Autodesk Inventor part; units mm, degrees
ref_plane "YZ Plane" through (0, 0, 0) normal (1, 0, 0) x (0, 1, 0)
ref_plane "XZ Plane" through (0, 0, 0) normal (0, 1, 0) x (-1, 0, 0)
ref_plane "XY Plane" through (0, 0, 0) normal (0, 0, 1) x (1, 0, 0)
sketch "Sketch1" plane through (0, 0, 0) normal (0, 1, 0) x (-1, 0, 0)
  line L0 (30.48, 38.1) -> (-30.48, 38.1)
  line L1 (-30.48, 38.1) -> (-30.48, -38.1)
  line L2 (-30.48, -38.1) -> (30.48, -38.1)
  line L3 (30.48, -38.1) -> (30.48, 38.1)
  point P0 (0, 0)
  dimension "d0" = 76.2
  dimension "d1" = 60.96
  dimension "d2" = 38.1
  dimension "d3" = 30.48
extrude "Extrusion1" add sketch "Sketch1" along normal blind 25.4
sketch "Sketch2" plane through (0, 25.4, 0) normal (0, 1, 0) x (1, 0, 0)
  line L0 (-28.8925, 36.5125) -> (28.8925, 36.5125)
  line L1 (28.8925, 36.5125) -> (28.8925, -36.5125)
  line L2 (28.8925, -36.5125) -> (-28.8925, -36.5125)
  line L3 (-28.8925, -36.5125) -> (-28.8925, 36.5125)
  point P0 (0, 0)
  dimension "d6" = 73.025
  dimension "d7" = 57.785
  dimension "d8" = 36.5125
  dimension "d9" = 28.8925
extrude "Extrusion2" cut sketch "Sketch2" against normal blind 19.05
chamfer "Chamfer1" distance 0.7937 angle 45 8 edges at (0, 0, 38.1) (30.48, 0, 0) (0, 0, -38.1) (-30.48, 0, 0) (30.48, 12.7, 38.1) (-30.48, 12.7, 38.1) (30.48, 12.7, -38.1) (-30.48, 12.7, -38.1)
sketch "Sketch3" plane through (0, 6.35, 0) normal (0, 1, 0) x (1, 0, 0)
  circle A0 centre (-22.86, 30.48) radius 1.9304
  circle A1 centre (22.86, 30.48) radius 1.9304
  circle A2 centre (-22.86, -30.48) radius 1.9304
  circle A3 centre (22.86, -30.48) radius 1.9304
  line L0 (-28.8925, -36.5125) -> (-28.8925, 36.5125)
  line L1 (-28.8925, 36.5125) -> (28.8925, 36.5125)
  line L2 (0, 0) -> (0, 32.9664)
  line L3 (0, 0) -> (-24.0434, 0)
  line L4 (0, 0) -> (25.6064, 0)
  line L5 (0, 0) -> (0, -31.6413)
  dimension "d15" = 3.8608
  dimension "d16" = 3.8608
  dimension "d17" = 3.8608
  dimension "d18" = 3.8608
  dimension "d21" = 30.48
  dimension "d22" = 22.86
  dimension "d23" = 22.86
  dimension "d24" = 30.48
  dimension "d25" = 22.86
  dimension "d26" = 30.48
  dimension "d27" = 22.86
  dimension "d28" = 30.48
extrude "Extrusion3" cut sketch "Sketch3" against normal blind 6.35
sketch "Sketch4" plane through (0, 0, 0) normal (0, -1, 0) x (1, 0, 0)
  circle A0 centre (-22.86, 30.48) radius 5.08
  line L0 (0, 0) -> (-26.2361, 0)
  line L1 (-26.2361, 0) -> (0, 0)
  line L2 (0, 0) -> (0, 35.0708)
  line L3 (0, 0) -> (27.0223, 0)
  line L4 (0, 0) -> (0, -33.193)
  circle A1 centre (22.86, 30.48) radius 5.08
  circle A2 centre (-22.86, -30.48) radius 5.08
  circle A3 centre (22.86, -30.48) radius 1.9304
  circle A4 centre (22.86, -30.48) radius 5.08
  dimension "d31" = 10.16
  dimension "d32" = 22.86
  dimension "d33" = 30.48
  dimension "d34" = 10.16
  dimension "d35" = 22.86
  dimension "d36" = 30.48
  dimension "d37" = 10.16
  dimension "d38" = 10.16
  dimension "d39" = 30.48
  dimension "d40" = 22.86
extrude "Extrusion4" cut sketch "Sketch4" against normal blind 3.175
properties part number "Enclosure Rev A"
Check sheet for the modelled part. Datum: model origin and axes. Units: mm. A direction names the side the tool comes from. Coordinates: 2 decimals unless noted, no trailing zeros. Loops run counter-clockwise (first coordinate to the right, second up) from the corner with the lowest first, then second, coordinate; pieces in that order, holes last. Notation, with made-up numbers: (33.5, 50.5) -> (70.5, 50.5) arc R20 cw to (70.5, 82.5) -> close; hole circle Ø8 at (-1.5, -7). An arc over 180 degrees is marked (long way). Write item = value, one per line. Start each with the question number.
1. Draft check along X on faces 1 (the flat face through (0, 13, -38.1)), 2 (the flat face through (30.48, 13, 1)), 3 (the flat face through (23, 3.175, -33)). Enter one of: released by +X, released by -X, zero draft, split by the parting line, or undercut.
2. Section check D-D on x = 12.5. Record the cut outline in (y, z).
3. Depth check by flat-ended pin: P1, Ø2, axis at x = -16, z = 15, coming from the +Y side; P2, Ø3.5, axis at x = -22.86, z = -30.48, coming from the +Y side; P3, Ø8, axis at x = -22.86, z = -30.48, coming from the -Y side (3 decimals). Enter the tip coordinate at first touch or a pass-through.
4. Tool access check on faces 4 (the cylindrical face through (18.83, 1.57, 27.39)), 5 (the flat face through (28.892, 16, -1)), 6 (the flat face through (0, 25.4, 37)). Record the directions out of +Z, -Z, +X, -X, +Y, -Y that give a thin tool (end or side, any length) a straight path to the whole face; none if there is none.
5. Section check A-A on x = 22.86. Give the number of separate pieces and of enclosed holes in the cut face, then the cut area to 3 significant figures.
6. Section check C-C on y = 20.5. Record the cut outline in (x, z).
7. Material ranges on line 1 (Z direction, x = 22.86, y = 3.9); line 2 (Z direction, x = -22.86, y = 1.5); line 3 (X direction, y = 4.4, z = 30.48), recorded low to high.
Responses:
q1.face_1 = zero draft
q1.face_2 = released by +X
q1.face_3 = undercut
q2.outline = (0, -37.31) -> (0.79, -38.1) -> (25.4, -38.1) -> (25.4, -36.51) -> (6.35, -36.51) -> (6.35, 36.51) -> (25.4, 36.51) -> (25.4, 38.1) -> (0.79, 38.1) -> (0, 37.31) -> close
q3.P1 = 6.35
q3.P2 = through
q3.P3 = 3.175
q4.face_4 = -Y
q4.face_5 = +Y
q4.face_6 = +Z, -Z, +X, -X, +Y
q5.separate_pieces = 3
q5.enclosed_holes = 0
q5.area = 455 mm2
q6.outline = (-30.48, -37.31) -> (-29.69, -38.1) -> (29.69, -38.1) -> (30.48, -37.31) -> (30.48, 37.31) -> (29.69, 38.1) -> (-29.69, 38.1) -> (-30.48, 37.31) -> close; hole (-28.89, -36.51) -> (28.89, -36.51) -> (28.89, 36.51) -> (-28.89, 36.51) -> close
q7.line_1 = -38.1 to -32.41, -28.55 to 28.55, 32.41 to 38.1
q7.line_2 = -38.1 to -35.56, -25.4 to 25.4, 35.56 to 38.1
q7.line_3 = -30.48 to -24.79, -20.93 to 20.93, 24.79 to 30.48
